from build123d import *

# Parameters (mm, degrees)
F0_R     = 3.175
F0_R_2   = 3.96875
F1_DEPTH = 3.175
F2_R     = 7.9375


with BuildPart() as f1:
    # F0 (on Top) → F1 (new body)
    with BuildSketch(Plane.XY):
        with BuildLine():
            ThreePointArc((0.2834821429, -7.9324362036), (5.7120069047, -5.5115227815), (7.9375, 0))
            ThreePointArc((7.9375, 0), (5.7120069047, 5.5115227815), (0.2834821429, 7.9324362036))
            ThreePointArc((0.2834821429, 7.9324362036), (-7.9375, 0), (0.2834821429, -7.9324362036))
        make_face()
        Circle(F0_R, mode=Mode.SUBTRACT)
        with BuildLine():
            ThreePointArc((0.2834821429, -7.9324362036), (-7.9375, 0), (0.2834821429, 7.9324362036))
            Line((0.2834821429, 7.9324362036), (-44.1098214286, 9.5189234444))
            ThreePointArc((-44.1098214286, 9.5189234444), (-37.9213417577, 6.9355783144), (-34.968992794, 0.9144))
            Line((-34.968992794, 0.9144), (-33.9975998101, -9.157542126))
            Line((-33.9975998101, -9.157542126), (0.2834821429, -7.9324362036))
        make_face()
        with BuildLine():
            ThreePointArc((-34.968992794, 0.9144), (-37.9213417577, 6.9355783144), (-44.1098214286, 9.5189234444))
            ThreePointArc((-44.1098214286, 9.5189234444), (-50.7267940031, 7.1643200684), (-53.931007206, 0.9144))
            ThreePointArc((-53.931007206, 0.9144), (-51.3855783284, -6.5286582275), (-44.1098214693, -9.5189234458))
            ThreePointArc((-44.1098214693, -9.5189234458), (-37.5955917285, -6.6138273524), (-34.925, 0))
            ThreePointArc((-34.925, 0), (-34.9360045555, 0.4577288296), (-34.968992794, 0.9144))
        make_face()
        with Locations((-44.45, 0)):
            Circle(F0_R, mode=Mode.SUBTRACT)
        with BuildLine():
            Line((-28.9011481822, -62.000384), (-33.9975998101, -9.157542126))
            Line((-33.9975998101, -9.157542126), (-44.1098214693, -9.5189234458))
            ThreePointArc((-44.1098214693, -9.5189234458), (-51.3855783284, -6.5286582275), (-53.931007206, 0.9144))
            Line((-53.931007206, 0.9144), (-59.9988518178, -62.000384))
            ThreePointArc((-59.9988518178, -62.000384), (-44.45, -47.879), (-28.9011481822, -62.000384))
        make_face()
        with Locations((-44.45, -20.6502)):
            Circle(F0_R, mode=Mode.SUBTRACT)
        with BuildLine():
            Line((-44.1098214693, -9.5189234458), (-33.9975998101, -9.157542126))
            Line((-33.9975998101, -9.157542126), (-34.968992794, 0.9144))
            ThreePointArc((-34.968992794, 0.9144), (-34.9360045555, 0.4577288296), (-34.925, 0))
            ThreePointArc((-34.925, 0), (-37.5955917285, -6.6138273524), (-44.1098214693, -9.5189234458))
        make_face()
        with BuildLine():
            ThreePointArc((-28.829, -63.5), (-28.847047471, -62.7493247194), (-28.9011481822, -62.000384))
            ThreePointArc((-28.9011481822, -62.000384), (-44.45, -47.879), (-59.9988518178, -62.000384))
            ThreePointArc((-59.9988518178, -62.000384), (-45.2006752806, -79.102952529), (-28.829, -63.5))
        make_face()
        with Locations((-44.45, -63.5)):
            Circle(F0_R_2, mode=Mode.SUBTRACT)
    extrude(amount=F1_DEPTH)

    # F2
    f2_edges = [f1.edges().sort_by_distance(p)[0] for p in [
        (-33.9976, -9.157542, 1.5875),
    ]]
    fillet(f2_edges, radius=F2_R)


solid = f1.part
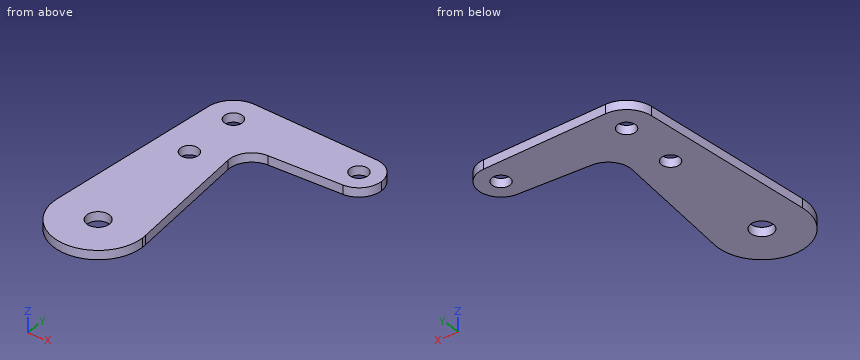
Geometry check sheet. Reference: the model listing, model coordinates, mm. Coordinates: 2 decimals unless noted, no trailing zeros. Loops run counter-clockwise (first coordinate to the right, second up) from the corner with the lowest first, then second, coordinate; pieces in that order, holes last. Notation, with made-up numbers: (1.25, 1.5) - (18.25, 1.5) arc R23 ccw to (18.25, 24.5) - close; hole circle Ø3 at (20.5, -29). An arc over 180 degrees is marked (long way). Use one line per item in the form item = value. Start each with the question number.
Item 1: Section check D-D, the plane x = -21. Enter the section's corners in (y, z) (3 decimals), and give its area (3 significant figures).
Item 2: Thickness scan on probe 1 along Y at (x, z) = (-44.45, 2.55) (3 decimals); probe 2 along Y at (x, z) = (1, 1.1); probe 3 along X at (y, z) = (-62, 2.7). Record the ranges inside material, lowest first.
Item 3: Gauge pin test, flat ends, axial feed: pin 1 (5 mm diameter, centred on x = -26.5, y = -46.5, fed in from +Z); pin 2 (1.5 mm diameter, centred on y = -64.5, z = 1, fed in from +X); pin 3 (1 mm diameter, centred on y = -61, z = 0.5, fed in from +X). Record the tip position at first contact, or that the pin passes through.
Item 4: Section check C-C, the plane y = -18.5. Enter the section's corners in (x, z) (3 decimals), and give its area (3 significant figures).
Item 5: Section check A-A, the plane y = -65. Enter the section's corners in (x, z) (3 decimals), and give its area (3 significant figures).
Item 6: Section check B-B, the plane z = 2.1. Give the number of separate pieces and of enclosed holes in the cut face, and give its area (3 significant figures).
Computed:
q1.outline = (-8.693, 0) - (8.693, 0) - (8.693, 3.175) - (-8.693, 3.175) - close
q1.area = 55.2 mm2
q2.probe_1 = -79.121 to -67.469, -59.531 to -23.825, -17.475 to -3.175, 3.175 to 9.525
q2.probe_2 = -7.87 to -3.01, 3.01 to 7.87
q2.probe_3 = -60 to -48.12, -40.78 to -28.9
q3.pin_1 = through
q3.pin_2 = -28.83
q3.pin_3 = -28.95
q4.outline = (-55.803, 0) - (-46.786, 0) - (-46.786, 3.175) - (-55.803, 3.175) - close; (-42.114, 0) - (-33.097, 0) - (-33.097, 3.175) - (-42.114, 3.175) - close
q4.area = 57.3 mm2
q5.outline = (-59.999, 0) - (-48.124, 0) - (-48.124, 3.175) - (-59.999, 3.175) - close; (-40.776, 0) - (-28.901, 0) - (-28.901, 3.175) - (-40.776, 3.175) - close
q5.area = 75.4 mm2
q6.separate_pieces = 1
q6.enclosed_holes = 4
q6.area = 2,710 mm2
